from build123d import *

# Parameters (mm, degrees)
SKETCH1_W           = 105
SKETCH1_H           = 65
BOSS_EXTRUDE1_DEPTH = 6
SKETCH3_W           = 54.9
SKETCH3_H           = 65
BOSS_EXTRUDE3_DEPTH = 1.9
SKETCH4_W           = 2.4
SKETCH4_H           = 24.2
SKETCH4_H_2         = 39.7
BOSS_EXTRUDE4_DEPTH = 3.1


with BuildPart() as part:
    # Sketch1 → Boss-Extrude1 (new body)
    with BuildSketch(Plane(origin=(0, 0, 0), x_dir=(1, 0, 0), z_dir=(0, 1, 0))):
        Rectangle(SKETCH1_W, SKETCH1_H)
    extrude(amount=BOSS_EXTRUDE1_DEPTH)

    # Sketch3 → Boss-Extrude3 (add)
    with BuildSketch(Plane.XZ):
        with Locations((-11.75, 0)):
            Rectangle(SKETCH3_W, SKETCH3_H)
    extrude(amount=BOSS_EXTRUDE3_DEPTH)

    # Sketch4 → Boss-Extrude4 (add)
    with BuildSketch(Plane.XZ.offset(1.9)):
        with Locations((-34.7, 15.1)):
            Rectangle(SKETCH4_W, SKETCH4_H)
        with Locations((9.453936311, 7.35)):
            Rectangle(SKETCH4_W, SKETCH4_H_2)
    extrude(amount=BOSS_EXTRUDE4_DEPTH)


solid = part.part
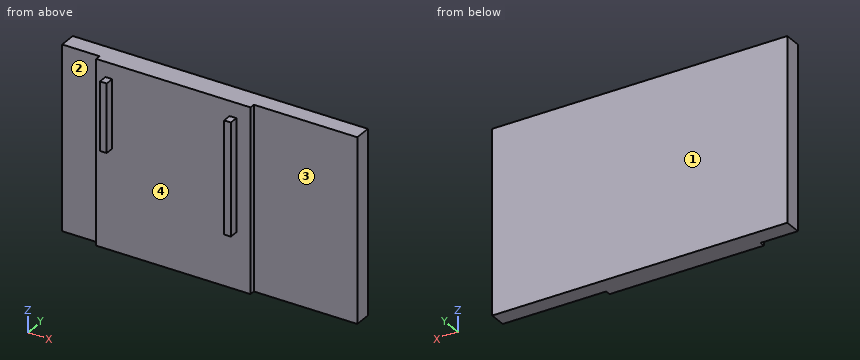
Verification items for the finished model (mm, model axes). Face numbers are marked on the shaded views. A direction names the side the tool comes from. Round coordinates to 2 decimals unless told otherwise and drop trailing zeros. Order: outer loops, then holes, each group sorted by start corner. A loop starts at its lowest first (then second) coordinate and runs counter-clockwise, first axis right, second up.
1. Go/stop test with flat-tipped pins: P1, Ø2.5, axis at x = 10, y = -3.5, coming from the -Z side; P2, Ø3.5, axis at y = -3, z = 18, coming from the +X side; P3, Ø3.5, axis at y = -2.5, z = 15, coming from the -X side. Record where each tip stops, or that it passes through.
Final values:
P1: stops at z = -12.5
P2: stops at x = 15.7
P3: stops at x = -39.2
2. Section check D-D on x = 31.5. Record the cut outline in (y, z).
Final values:
outline: (0, -32.5) - (6, -32.5) - (6, 32.5) - (0, 32.5) - close
3. Thickness scan on L1, parallel to X at y = -2.5, z = 18; L2, parallel to Y at x = 16, z = 28; L3, parallel to Y at x = -32.5, z = 26. Record the ranges inside material, lowest first.
Final values:
L1: x = -35.9 to -33.5, 8.25 to 10.65
L2: y = 0 to 6
L3: y = -1.9 to 6
4. Section check A-A on z = 2. Record the cut outline in (x, y).
Final values:
outline: (-52.5, 0) - (-39.2, 0) - (-39.2, -1.9) - (8.25, -1.9) - (8.25, -5) - (10.65, -5) - (10.65, -1.9) - (15.7, -1.9) - (15.7, 0) - (52.5, 0) - (52.5, 6) - (-52.5, 6) - close
5. Release check for a two-part mould opening along X. For the marked faces 3 and 4 record: +X half, -X half, draft (parallel to the pull), parting line (faces both ways), or undercut.
Final values:
face 3: draft
face 4: undercut
6. Section check B-B on x = 12. Record the cut outline in (y, z), then the cut area to 4 significant figures.
Final values:
outline: (-1.9, -32.5) - (6, -32.5) - (6, 32.5) - (-1.9, 32.5) - close
area: 513.5 mm2
7. Section check C-C on z = -26. Record the cut outline in (x, y), then the cut area to 3 significant figures.
Final values:
outline: (-52.5, 0) - (-39.2, 0) - (-39.2, -1.9) - (15.7, -1.9) - (15.7, 0) - (52.5, 0) - (52.5, 6) - (-52.5, 6) - close
area: 734 mm2
8. Access from +Z, -Z, +X, -X, +Y, -Y to the whole of each face (thin tool, end or side, straight path). Record for the marked faces 1 and 2.
Final values:
face 1: +Z, -Z, +X, -X, +Y
face 2: +Z, -Z, -X, -Y
